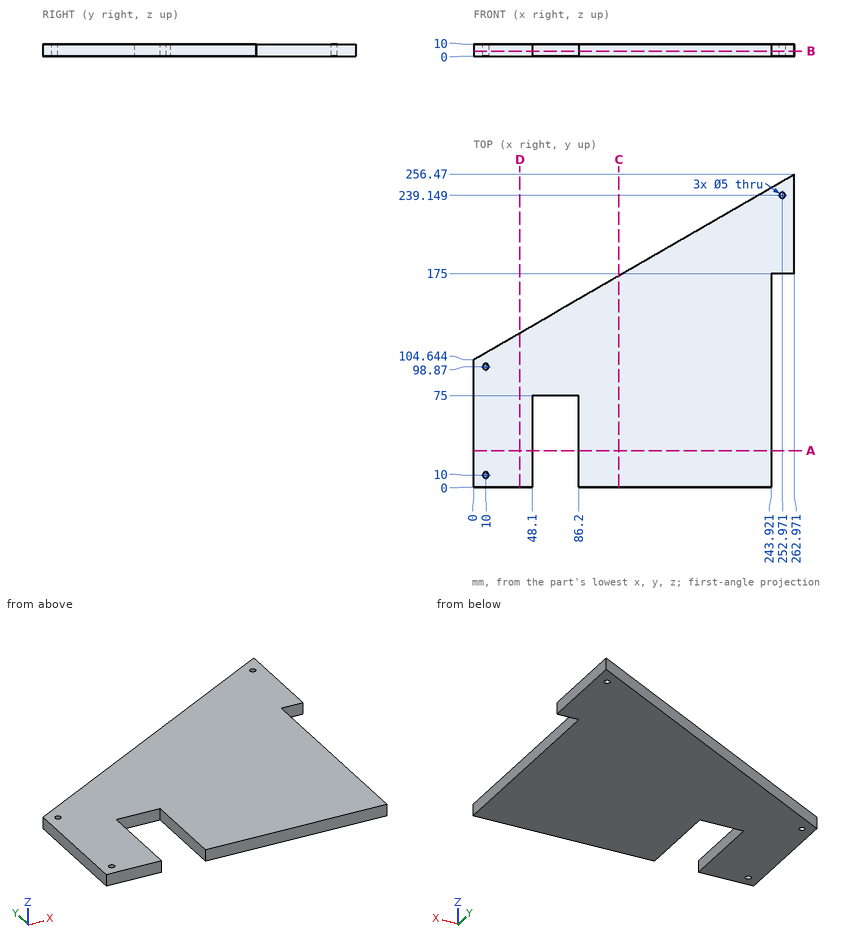
Study the drawing (mm; zero at the part's minimum x, y, z) and answer. Round coordinates to 2 decimals unless told otherwise and drop trailing zeros. Loops run counter-clockwise (first coordinate to the right, second up) from the corner with the lowest first, then second, coordinate; pieces in that order, holes last. Notation, with made-up numbers: (8, -19) - (55, -19) arc R7 ccw to (55, -14) - close; hole circle Ø11 at (68.25, 25.25). An arc over 180 degrees is marked (long way). Use one line per item in the form item = value. Start each with the question number.
1. The part is cut by section C-C on x = 119. Determine the outline of the cut face in (y, z), then the cut area to 3 significant figures.
2. Consider line 1 (X direction, y = 29.5, z = 2.5); line 2 (Y direction, x = 10, z = 3) (1 decimal); line 3 (X direction, y = 101.5, z = 4). Determine where each line is inside the solid, lowest interval first. Write a range as [from, to].
3. The part is cut by section D-D on x = 38. Determine the outline of the cut face in (y, z).
4. The part is cut by section A-A on y = 30. Determine the outline of the cut face in (x, z), then the cut area to 3 significant figures.
5. The part is cut by section B-B on z = 4.25. Determine the outline of the cut face in (x, y).
6. Given pin 1 Ø5 at (y, z) = (51.5, 3) entering from +X; pin 2 Ø4.5 at (x, y) = (10, 10) entering from -Z; pin 3 Ø3 at (x, z) = (65.5, 3.5) entering from -Y; pin 4 Ø3 at (x, z) = (253.5, 7) entering from -Y, each flat-ended and moving along its own axis, determine where each tip first touches the part or whether it passes through.
Geometry check:
q1.outline = (0, 0) - (173.35, 0) - (173.35, 10) - (0, 10) - close
q1.area = 1,730 mm^2
q2.line_1 = [0, 48.1], [86.2, 243.92]
q2.line_2 = [0, 7.5], [12.5, 96.4], [101.4, 110.4]
q2.line_3 = [0, 243.92]
q3.outline = (0, 0) - (126.58, 0) - (126.58, 10) - (0, 10) - close
q4.outline = (0, 0) - (48.1, 0) - (48.1, 10) - (0, 10) - close; (86.2, 0) - (243.92, 0) - (243.92, 10) - (86.2, 10) - close
q4.area = 2,060 mm^2
q5.outline = (0, 0) - (48.1, 0) - (48.1, 75) - (86.2, 75) - (86.2, 0) - (243.92, 0) - (243.92, 175) - (262.97, 175) - (262.97, 256.47) - (0, 104.64) - close; hole circle Ø5 at (10, 10); hole circle Ø5 at (10, 98.87); hole circle Ø5 at (252.97, 239.15)
q6.pin_1 = 243.92
q6.pin_2 = through
q6.pin_3 = 75
q6.pin_4 = 175
